Part print with two shaded views. Sizes in mm from the minimum x, y, z corner. A direction names the side the tool comes from. Coordinates: 2 decimals unless noted, no trailing zeros. Write each loop counter-clockwise with the first axis right and the second up, starting at its lowest first coordinate (ties: lowest second). Pieces come first, ordered by that corner, then holes. Notation, with made-up numbers: (-5, -38.5) - (27, -38.5) arc R26 cw to (27, -20.5) - close; hole circle Ø7 at (80.25, -24). An arc over 180 degrees is marked (long way). Answer in a Markdown table with one row per item. Add a question column.
Q1. 3-axis set-ups, long thin cutter, end or side, ignore diameter. For the marked faces 4 and 5: which of +Z, -Z, +X, -X, +Y, -Y reach the whole face in a straight line?
Q2. Drill centre lines: line 1 along Z through (x, y) = (17, 7); line 2 along X through (y, z) = (5, 7.5); line 3 along X through (y, z) = (6, 12.5) (1 decimal). Where is each one in solid material? Low to high. Write a range as from..to.
Q3. Band-saw the part on B-B (y = 7.5). List the corners of the cut face in (x, z).
Q4. Two-plate mould, pull along Y, no slides. Class the marked faces 1, 2 and 3: +Y half, -Y half, draft (parallel to the pull), parting line (faces both ways), or undercut.
Q5. Band-saw the part on C-C (z = 9.5). List the corners of the cut face in (x, y).
Q6. Pin check, flat tips, straight feed: pin 1 (6 mm diameter, centred on x = 6, z = 4.5, fed in from -Y); pin 2 (4 mm diameter, centred on y = 4, z = 9, fed in from +X); pin 3 (3 mm diameter, centred on x = 19.46, y = 7.5, fed in from +Z). Stop position of each tip, or through.
Q7. Band-saw the part on A-A (x = 6). List the corners of the cut face in (y, z), and give its area (3 significant figures).
Q8. Band-saw the part on D-D (y = 11.5). List the corners of the cut face in (x, z).
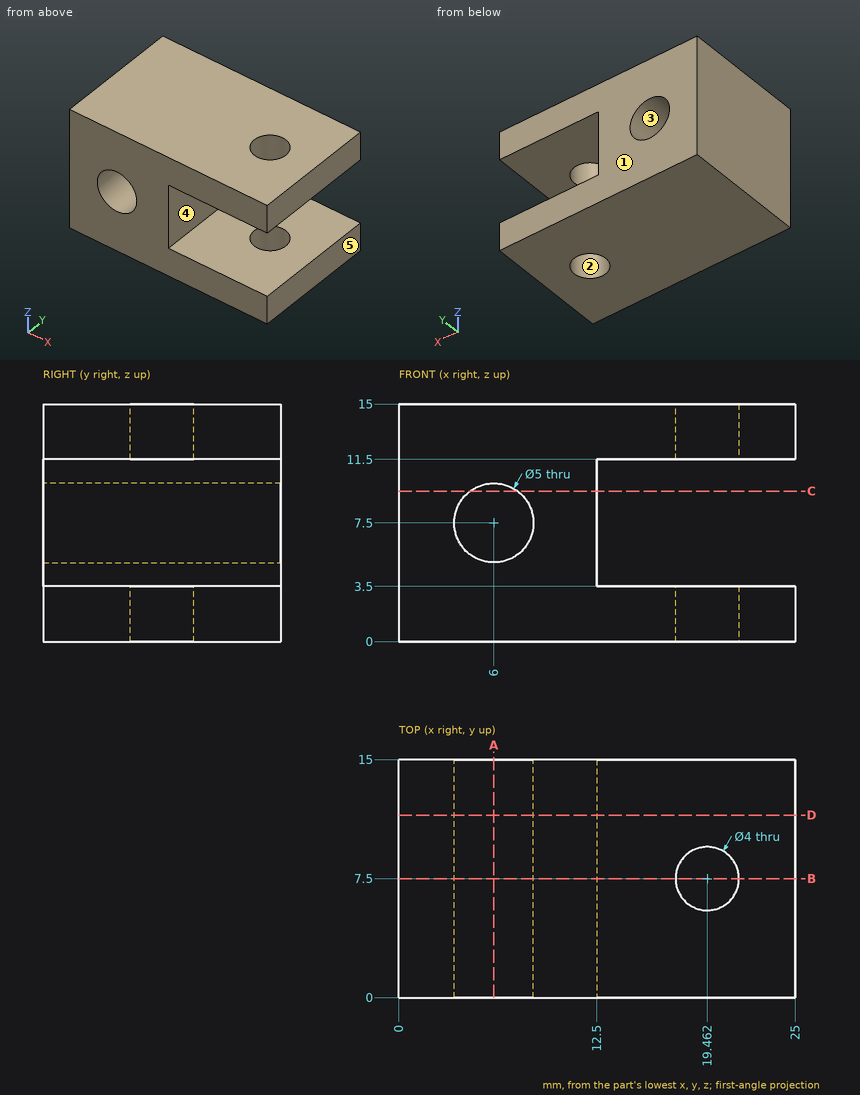
Checked values:
| question | item | result |
|---|---|---|
| 1 | face 4 | +X, +Y, -Y |
| 1 | face 5 | +Z, -Z, +X, +Y, -Y |
| 2 | line 1 | z = 0..3.5, 11.5..15 |
| 2 | line 2 | x = 0..3.5, 8.5..12.5 |
| 2 | line 3 | x = 0..18.1, 20.8..25 |
| 3 | outline | (0, 0) - (17.46, 0) - (17.46, 3.5) - (12.5, 3.5) - (12.5, 11.5) - (17.46, 11.5) - (17.46, 15) - (0, 15) - close; (21.46, 0) - (25, 0) - (25, 3.5) - (21.46, 3.5) - close; (21.46, 11.5) - (25, 11.5) - (25, 15) - (21.46, 15) - close; hole circle Ø5 at (6, 7.5) |
| 4 | face 1 | +Y half |
| 4 | face 2 | undercut |
| 4 | face 3 | draft |
| 5 | outline | (0, 0) - (4.5, 0) - (4.5, 15) - (0, 15) - close; (7.5, 0) - (12.5, 0) - (12.5, 15) - (7.5, 15) - close |
| 6 | pin 1 | stops at y = 0 |
| 6 | pin 2 | stops at x = 12.5 |
| 6 | pin 3 | passes through |
| 7 | outline | (0, 0) - (15, 0) - (15, 5) - (0, 5) - close; (0, 10) - (15, 10) - (15, 15) - (0, 15) - close |
| 7 | area | 150 mm² |
| 8 | outline | (0, 0) - (25, 0) - (25, 3.5) - (12.5, 3.5) - (12.5, 11.5) - (25, 11.5) - (25, 15) - (0, 15) - close; hole circle Ø5 at (6, 7.5) |
